Design review of the part built by this model. Coordinates are the model's own, in mm. Coordinates: 2 decimals unless noted, no trailing zeros. Write each loop counter-clockwise with the first axis right and the second up, starting at its lowest first coordinate (ties: lowest second). Pieces come first, ordered by that corner, then holes.
Q1. Add section A-A, the plane y = 213.5. Give the boundary of the cut face in (x, z), plus the area to 3 significant figures.
Q2. The part is to be moulded in two halves that separate along X. For faces 1 (the face through (38.5, 222, 2)), 2 (the face through (-66.5, 116, 2)), 3 (the face through (3, 93, 4.826)), 4 (the face through (-31.5, 222, 2)), say which applies: +X half, -X half, draft (parallel to the pull), parting line (faces both ways), or undercut.
Q3. To check wall thickness, follow probe 1 along X at (y, z) = (152.5, 0.4); probe 2 along X at (y, z) = (172.5, 2.9); probe 3 along Y at (x, z) = (6, 3.05). State the ranges of each line that lie inside material, in increasing order.
from build123d import *

# Parameters (mm, degrees)
F0_W      = 140
F0_H      = 110
F0_W_2    = 35
F0_H_2    = 25
F1_DEPTH  = 4.826
F2_W      = 31.75
F2_H      = 31.75
F2_W_2    = 25.4
F2_H_2    = 25.4
F3_DEPTH  = 120
F4_W      = 6
F4_H      = 31.75
F4_W_2    = 2.825
F4_H_2    = 25.4
F5_DEPTH  = 110
F6_R      = 3
F7_DEPTH  = 10
F8_W      = 25.4
F8_H      = 25.4
F8_W_2    = 15.874
F8_H_2    = 15.874
F9_DEPTH  = 20
F11_DEPTH = 152
F12_W     = 120
F12_H     = 31.75
F13_DEPTH = 140.0010001


with BuildPart() as f1:
    # F0 (on Top) → F1 (new body)
    with BuildSketch(Plane.XY):
        with Locations((3.5, 55)):
            Rectangle(F0_W, F0_H)
        with BuildLine():
            Line((-66.5, 210), (-66.5, 110))
            Line((-66.5, 110), (73.5, 110))
            Line((73.5, 110), (73.5, 210))
            Line((73.5, 210), (38.5, 210))
            add(Edge.make_bspline(
                [(-31.5, 210), (-31.5, 178), (-26.1927577262, 110.7427430843), (33.1927577262, 110.7427430843), (38.5, 178), (38.5, 210)],
                knots=[0, 0, 0, 0, 0.3861272069, 0.6138727931, 1, 1, 1, 1], degree=3))
            Line((-31.5, 210), (-66.5, 210))
        make_face()
        with Locations((-49, 222.5)):
            Rectangle(F0_W_2, F0_H_2)
        with Locations((56, 222.5)):
            Rectangle(F0_W_2, F0_H_2)
    extrude(amount=F1_DEPTH)

    # F2 (on face) → F3 (join)
    with BuildSketch(Plane.XZ):
        with Locations((-50.625, -15.875)):
            Rectangle(F2_W, F2_H)
        with Locations((-50.625, -15.875)):
            Rectangle(F2_W_2, F2_H_2, mode=Mode.SUBTRACT)
        with Locations((57.625, -15.875)):
            Rectangle(F2_W, F2_H)
        with Locations((57.625, -15.875)):
            Rectangle(F2_W_2, F2_H_2, mode=Mode.SUBTRACT)
    extrude(amount=-F3_DEPTH)

    # F4 (on face) → F5 (join)
    with BuildSketch(Plane(origin=(0, 120, 0), x_dir=(-1, 0, 0), z_dir=(0, 1, 0))):
        with Locations((63.5, -15.875)):
            Rectangle(F4_W, F4_H)
        with Locations((-68.9125, -15.875)):
            Rectangle(F4_W_2, F4_H_2)
        Polygon((-67.5, 0), (-73.5, 0), (-73.5, -31.75), (-70.325, -31.75), (-67.5, -31.75), (-67.5, -28.575), (-70.325, -28.575), (-70.325, -3.175), (-67.5, -3.175), align=None)
    extrude(amount=F5_DEPTH)

    # F6 (on face) → F7 (cut)
    with BuildSketch(Plane.YZ.offset(-34.75)):
        with Locations((60, -10)):
            Circle(F6_R)
    extrude(amount=-F7_DEPTH, mode=Mode.SUBTRACT)

    # F8 (on face) → F9 (join, symmetric)
    with BuildSketch(Plane.XZ):
        with Locations((-50.625, -15.875)):
            Rectangle(F8_W, F8_H)
        with Locations((-50.625, -15.875)):
            Rectangle(F8_W_2, F8_H_2, mode=Mode.SUBTRACT)
        with Locations((57.625, -15.875)):
            Rectangle(F8_W, F8_H)
        with Locations((57.625, -15.875)):
            Rectangle(F8_W_2, F8_H_2, mode=Mode.SUBTRACT)
    extrude(amount=F9_DEPTH, both=True)

    # F10 (on face) → F11 (cut)
    with BuildSketch(Plane(origin=(-66.5, 0, 0), x_dir=(0, -1, 0), z_dir=(-1, 0, 0))):
        with BuildLine():
            ThreePointArc((-180, -20), (-177.1715728753, -18.8284271247), (-176, -16))
            ThreePointArc((-176, -16), (-177.1715728753, -13.1715728753), (-180, -12))
            Line((-180, -12), (-180, -16))
            Line((-180, -16), (-180, -20))
        make_face()
        with BuildLine():
            Line((-180, -16), (-180, -12))
            ThreePointArc((-180, -12), (-184, -16), (-180, -20))
            Line((-180, -20), (-180, -16))
        make_face()
        with BuildLine():
            ThreePointArc((-180, -20), (-184, -16), (-180, -12))
            Line((-180, -12), (-230, -12))
            Line((-230, -12), (-230, -20))
            Line((-230, -20), (-180, -20))
        make_face()
    extrude(amount=-F11_DEPTH, mode=Mode.SUBTRACT)

    # F12 (on face) → F13 (cut, through all)
    with BuildSketch(Plane(origin=(-66.5, 0, 0), x_dir=(0, -1, 0), z_dir=(-1, 0, 0))):
        Polygon((-236.2957447767, 41.7925678194), (-236.2957447767, 0), (-235, 0), (-235, 4.826), (-120, 4.826), (-120, 41.7925678194), align=None)
        Polygon((-120, 64.1580745578), (-120, 41.7925678194), (11.4044835791, 41.7925678194), (11.4044835791, 0), (0, 0), (0, -31.75), (-120, -31.75), (-120, -61.878118664), (43.3997410536, -61.878118664), (43.3997410536, 64.1580745578), align=None)
        with Locations((-60, -15.875)):
            Rectangle(F12_W, F12_H)
        Polygon((11.4044835791, 41.7925678194), (-120, 41.7925678194), (-120, 4.826), (0, 4.826), (0, 0), (11.4044835791, 0), align=None)
        with BuildLine():
            Line((-120, 0), (-230, 0))
            Line((-230, 0), (-230, -12))
            Line((-230, -12), (-180, -12))
            ThreePointArc((-180, -12), (-176, -16), (-180, -20))
            Line((-180, -20), (-230, -20))
            Line((-230, -20), (-230, -31.75))
            Line((-230, -31.75), (-120, -31.75))
            Line((-120, -31.75), (-120, 0))
        make_face()
    extrude(amount=-F13_DEPTH, mode=Mode.SUBTRACT)


solid = f1.part
Here are the results:
1. outline: (-66.5, 0) - (-31.5, 0) - (-31.5, 4.83) - (-66.5, 4.83) - close; (38.5, 0) - (73.5, 0) - (73.5, 4.83) - (38.5, 4.83) - close
1. area: 338 mm2
2. face 1: undercut
2. face 2: -X half
2. face 3: draft
2. face 4: undercut
3. probe 1: x = -66.5 to -26.67, 33.67 to 73.5
3. probe 2: x = -66.5 to -29.71, 36.71 to 73.5
3. probe 3: y = 0 to 113.21
